Source: CAD feature listing. Evaluate the final solid. Frame: model axes, mm. Coordinates: 2 decimals unless noted, no trailing zeros. Write each loop counter-clockwise with the first axis right and the second up, starting at its lowest first coordinate (ties: lowest second). Pieces come first, ordered by that corner, then holes. Notation, with made-up numbers: (26.5, 1.25) - (39.5, 1.25) arc R17 cw to (39.5, 28.25) - close; hole circle Ø4 at (27, 53). An arc over 180 degrees is marked (long way). One line per item, written item: value.
Autodesk Inventor part; units mm, degrees
ref_plane "YZ Plane" through (0, 0, 0) normal (1, 0, 0) x (0, 1, 0)
ref_plane "XZ Plane" through (0, 0, 0) normal (0, 1, 0) x (-1, 0, 0)
ref_plane "XY Plane" through (0, 0, 0) normal (0, 0, 1) x (1, 0, 0)
sketch "스케치1" plane through (0, 0, 0) normal (0, 0, 1) x (1, 0, 0)
  line L0 (0, 45) -> (38.9711, 22.5)
  line L1 (38.9711, 22.5) -> (38.9711, -22.5)
  line L2 (38.9711, -22.5) -> (0, -45)
  line L3 (0, -45) -> (-38.9711, -22.5)
  line L4 (-38.9711, -22.5) -> (-38.9711, 22.5)
  line L5 (-38.9711, 22.5) -> (0, 45)
  line L6 (0, 50.7735) -> (43.9711, 25.3868)
  line L7 (43.9711, 25.3868) -> (43.9711, -25.3868)
  line L8 (43.9711, -25.3868) -> (0, -50.7735)
  line L9 (0, -50.7735) -> (-43.9711, -25.3868)
  line L10 (-43.9711, -25.3868) -> (-43.9711, 25.3868)
  line L11 (-43.9711, 25.3868) -> (0, 50.7735)
  circle A0 centre (-41.4711, 0) radius 2.5 construction
  circle A1 centre (-41.4711, 0) radius 2.6
  circle A2 centre (-20.7356, -35.9151) radius 2.6
  circle A3 centre (20.7356, -35.9151) radius 2.6
  circle A4 centre (41.4711, 0) radius 2.6
  circle A5 centre (20.7356, 35.9151) radius 2.6
  circle A6 centre (-20.7356, 35.9151) radius 2.6
  point P0 (0, 0)
  point P1 (0, 0)
  point P2 (-22.604, 37.7231)
  point P3 (-43.9711, 0.7141)
  point P4 (-43.9711, -0.7141)
  point P5 (-22.604, -37.7231)
  point P6 (-21.3671, -38.4372)
  point P7 (21.3671, -38.4372)
  point P8 (22.604, -37.7231)
  point P9 (43.9711, -0.7141)
  point P10 (43.9711, 0.7141)
  point P11 (22.604, 37.7231)
  point P12 (21.3671, 38.4372)
  point P13 (-21.3671, 38.4372)
  dimension "d0" = 45
  dimension "d1" = 5
  dimension "d2" = 5
  dimension "d3" = 5.2
  dimension "d6" = 360
extrude "돌출1" add sketch "스케치1" along normal blind 5 contours L5 A6 L11 L6 A5 L0 | L0 A5 L1 A4 L2 A3 L3 A2 L4 A1 L5 A6 | A5 L6 L7 A4 L1 L0 | L5 L4 A1 L10 L11 A6 | A4 L7 L8 A3 L2 L1 | L4 L3 A2 L9 L10 A1 | A3 L8 L9 A2 L3 L2
fillet "모깎기1" radius 1 12 edges at (-22.604, 37.7231, 2.5) (-21.3671, 38.4372, 2.5) (-43.9711, 0.7141, 2.5) (-43.9711, -0.7141, 2.5) (-22.604, -37.7231, 2.5) (-21.3671, -38.4372, 2.5) (21.3671, -38.4372, 2.5) (22.604, -37.7231, 2.5) (43.9711, -0.7141, 2.5) (43.9711, 0.7141, 2.5) (21.3671, 38.4372, 2.5) (22.604, 37.7231, 2.5)
sketch "스케치2" plane through (0, 0, 5) normal (0, 0, 1) x (1, 0, 0)
  circle A0 centre (0, 0) radius 26.325
  dimension "d11" = 52.65
extrude "돌출2" cut sketch "스케치2" against normal through all
sketch "스케치3" plane through (0, 0, 5) normal (0, 0, 1) x (1, 0, 0)
  circle A0 centre (0, 0) radius 26.325 construction
  circle A1 centre (0, 0) radius 29.75
  circle A2 centre (0, 29.75) radius 2
  circle A3 centre (-29.75, 0) radius 2
  circle A4 centre (0, -29.75) radius 2
  circle A5 centre (29.75, 0) radius 2
  dimension "d14" = 59.5
  dimension "d15" = 4
  dimension "d18" = 360
extrude "돌출3" add sketch "스케치3" along normal blind 4 contours A1 A5 | A1 A5 | A2 A1 | A1 A2 | A4 A1 | A1 A4 | A3 A1 | A1 A3
chamfer "모따기1" distance 1 angle 45 4 edges at (-31.75, 0, 9) (-2, 29.75, 9) (27.75, 0, 9) (-2, -29.75, 9)
properties part number "inner_top"
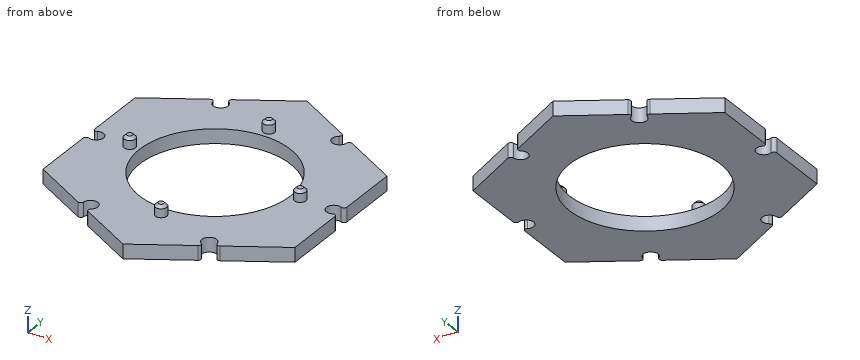
1) Section query C-C on x = -13. Output: boundary loops of the cut face in (y, z).
Values found:
outline: (-43.27, 0) - (-22.89, 0) - (-22.89, 5) - (-43.27, 5) - close; (22.89, 0) - (43.27, 0) - (43.27, 5) - (22.89, 5) - close
2) Contact query for flat-ended pins moving along their axis: P1, Ø6, axis at x = -41.47, y = 0, coming from the +Z side; P2, Ø4.5, axis at x = -20.74, y = -35.92, coming from the +Z side; P3, Ø2, axis at x = -32, z = 5, coming from the +Y side; P4, Ø1.5, axis at y = 2, z = 3.5, coming from the -X side. Output: stop coordinate, or through.
Values found:
P1: z = 5
P2: through
P3: y = 32.88
P4: x = -43.82
3) Material intervals for line 1 (Y direction, x = 0, z = 1.15) (1 decimal); line 2 (Z direction, x = -32, y = 24.5); line 3 (Y direction, x = -30, z = 6), sorted ascending.
Values found:
line 1: -50.8 to -26.3, 26.3 to 50.8
line 2: 0 to 5
line 3: -1.98 to 1.98
4) Section query D-D on z = 6.5. Output: boundary loops of the cut face in (x, y), then the cut area to 3 significant figures.
Values found:
outline: circle Ø4 at (-29.75, 0); circle Ø4 at (0, -29.75); circle Ø4 at (0, 29.75); circle Ø4 at (29.75, 0)
area: 50.3 mm2
5) Section query A-A on y = -16.5. Output: boundary loops of the cut face in (x, z).
Values found:
outline: (-43.97, 0) - (-20.51, 0) - (-20.51, 5) - (-43.97, 5) - close; (20.51, 0) - (43.97, 0) - (43.97, 5) - (20.51, 5) - close
